Job drawing, mm, ordinate dimensions from the low corner. One solid piece. A direction names the side the tool comes from. Round coordinates to 2 decimals unless told otherwise and drop trailing zeros. Order: outer loops, then holes, each group sorted by start corner. A loop starts at its lowest first (then second) coordinate and runs counter-clockwise, first axis right, second up. Notation, with made-up numbers: (17.25, 67.25) -> (51.25, 67.25) arc R24 cw to (51.25, 81.25) -> close; hole circle Ø10 at (84.25, 84). An arc over 180 degrees is marked (long way). Return JSON: item names as keys, results as strings. Group by question number.
Q1. Probe line 1 along Y through (x, z) = (24, 6.5) (3 decimals); line 2 along Y through (x, z) = (23.5, 3) (3 decimals); line 3 along X through (y, z) = (58.5, 1) (3 decimals). List the from-to ranges inside material, lowest first.
Q2. Flat gauge pins, fed straight in: pin 1 (3 mm diameter, centred on y = 49, z = 5, fed in from -X) (3 decimals); pin 2 (5 mm diameter, centred on y = 56.5, z = 4, fed in from +X) (3 decimals); pin 3 (5 mm diameter, centred on x = 29, z = 3, fed in from +Y) (3 decimals). Where does each tip first touch, or does it go through?
Q3. Which spindle directions (+Z, -Z, +X, -X, +Y, -Y) get a long thin tool onto all of the face, cutting with end or side? Do the marked faces 1, 2 and 3. Say none if no direction does.
Q4. Cut at B-B (x = 5.5). Write the cut outline in (y, z) (3 decimals).
Q5. Mould opens along X. For the marked faces 4 and 5 say: +X half, -X half, draft (parallel to the pull), parting line (faces both ways), or undercut.
Q6. Cut at A-A (y = 16.51). Write the cut outline in (x, z) (3 decimals).
Q7. Cut at D-D (x = 12). Write the cut outline in (y, z) (3 decimals), then the cut area to 3 significant figures.
Q8. Cut at C-C (z = 6.25). Write the cut outline in (x, y) (3 decimals), then the cut area to 3 significant figures.
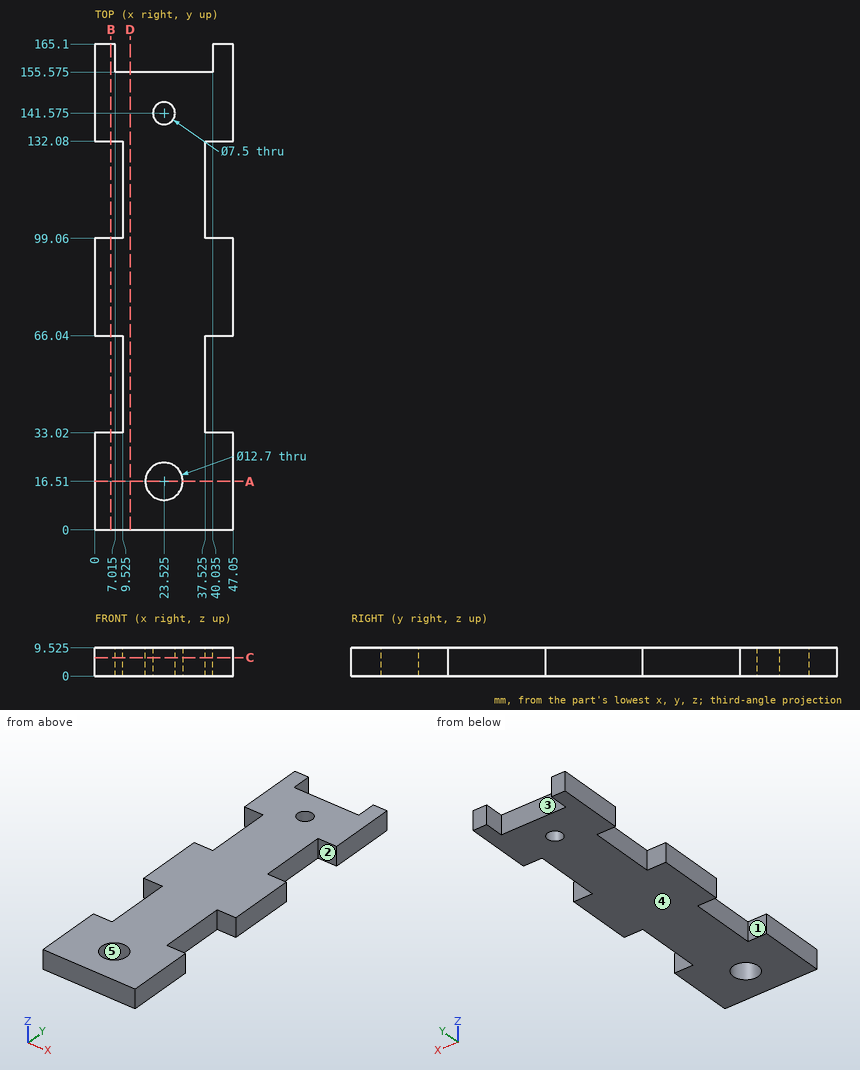
Solution:
{
 "1": {"line 1": "y = 0 to 10.178, 22.842 to 137.855, 145.295 to 155.575", "line 2": "y = 0 to 10.16, 22.86 to 137.825, 145.325 to 155.575", "line 3": "x = 9.525 to 37.525"},
 "2": {"pin 1": "stops at x = 9.525", "pin 2": "stops at x = 37.525", "pin 3": "stops at y = 155.575"},
 "3": {"face 1": "+Z, -Z, -X", "face 2": "+Z, -Z, +X", "face 3": "+Z, -Z, +Y"},
 "4": {"outline": "(0, 0) -> (33.02, 0) -> (33.02, 9.525) -> (0, 9.525) -> close; (66.04, 0) -> (99.06, 0) -> (99.06, 9.525) -> (66.04, 9.525) -> close; (132.08, 0) -> (165.1, 0) -> (165.1, 9.525) -> (132.08, 9.525) -> close"},
 "5": {"face 4": "draft", "face 5": "undercut"},
 "6": {"outline": "(0, 0) -> (17.175, 0) -> (17.175, 9.525) -> (0, 9.525) -> close; (29.875, 0) -> (47.05, 0) -> (47.05, 9.525) -> (29.875, 9.525) -> close"},
 "7": {"outline": "(0, 0) -> (155.575, 0) -> (155.575, 9.525) -> (0, 9.525) -> close", "area": "1,480 mm²"},
 "8": {"outline": "(0, 0) -> (47.05, 0) -> (47.05, 33.02) -> (37.525, 33.02) -> (37.525, 66.04) -> (47.05, 66.04) -> (47.05, 99.06) -> (37.525, 99.06) -> (37.525, 132.08) -> (47.05, 132.08) -> (47.05, 165.1) -> (40.035, 165.1) -> (40.035, 155.575) -> (7.015, 155.575) -> (7.015, 165.1) -> (0, 165.1) -> (0, 132.08) -> (9.525, 132.08) -> (9.525, 99.06) -> (0, 99.06) -> (0, 66.04) -> (9.525, 66.04) -> (9.525, 33.02) -> (0, 33.02) -> close; hole circle Ø12.7 at (23.525, 16.51); hole circle Ø7.5 at (23.525, 141.575)", "area": "6,020 mm²"}
}
